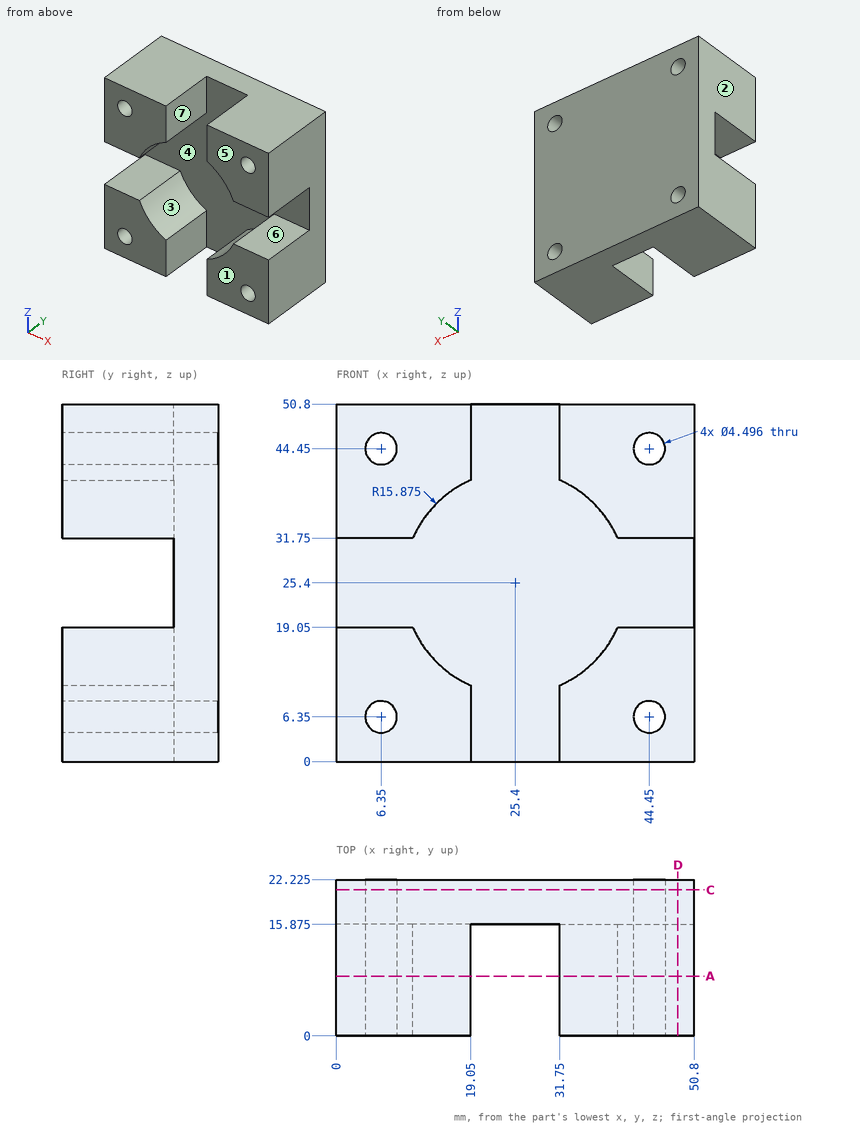
Geometry check sheet. Reference: drawing and pictorial views, mm from the part's lowest x, y, z. A direction names the side the tool comes from. Give positions to 0.01 mm unless a question says otherwise; leave off trailing zeros. Write each loop counter-clockwise with the first axis right and the second up, starting at its lowest first coordinate (ties: lowest second). Pieces come first, ordered by that corner, then holes.
Item 1: Cross-section at D-D (x = 48.5). Enter the section's corners in (y, z) (3 decimals).
Item 2: Gauge pin test, flat end, axial feed: pin 1 (2.5 mm diameter, centred on x = 6.35, z = 44.45, fed in from +Y). Record the tip position at first contact, or that the pin passes through.
Item 3: Scan lines: L1, parallel to Z at x = 44.45, y = 9; L2, parallel to Z at x = 44.45, y = 17.5. Record each from-to range of solid material in increasing order.
Item 4: Cross-section at C-C (y = 20.75). Enter the section's corners in (x, z).
Item 5: Cross-section at A-A (y = 8.5). Count the separate pieces of the cut face and the enclosed holes in it, and give its area (3 significant figures).
Item 6: Draft check along X on the marked faces 1, 2, 3 and 4. Enter one of: released by +X, released by -X, zero draft, split by the parting line, or undercut.
Item 7: Access from +Z, -Z, +X, -X, +Y, -Y to the whole of each face (thin tool, end or side, straight path). Record for the marked faces 5, 6 and 7.
Report:
1. outline: (0, 0) - (22.225, 0) - (22.225, 50.8) - (0, 50.8) - (0, 31.75) - (15.875, 31.75) - (15.875, 19.05) - (0, 19.05) - close
2. pin 1: passes through
3. L1: z = 0 to 4.1, 8.6 to 19.05, 31.75 to 42.2, 46.7 to 50.8
3. L2: z = 0 to 4.1, 8.6 to 42.2, 46.7 to 50.8
4. outline: (0, 0) - (50.8, 0) - (50.8, 50.8) - (0, 50.8) - close; hole circle Ø4.5 at (6.35, 6.35); hole circle Ø4.5 at (6.35, 44.45); hole circle Ø4.5 at (44.45, 6.35); hole circle Ø4.5 at (44.45, 44.45)
5. separate pieces: 4
5. enclosed holes: 4
5. area: 1,220 mm2
6. face 1: zero draft
6. face 2: released by -X
6. face 3: undercut
6. face 4: undercut
7. face 5: +Z, -Z, +X, -X, -Y
7. face 6: +X, -X, -Y
7. face 7: +Z, -Z, -Y
